```python
from build123d import *

# Parameters (mm, degrees)
SKETCH1_W           = 175.26
SKETCH1_H           = 12.7
BOSS_EXTRUDE1_DEPTH = 98.425
SKETCH2_W           = 5.08
SKETCH2_H           = 6.35
CUT_EXTRUDE1_DEPTH  = 216.567302483
CUT_EXTRUDE2_DEPTH  = 133.392550867
CUT_EXTRUDE3_DEPTH  = 133.392550867


with BuildPart() as part:
    # Sketch1 → Boss-Extrude1 (new, symmetric)
    with BuildSketch(Plane(origin=(0, 0, 0), x_dir=(0, 0, -1), z_dir=(1, 0, 0))):
        Rectangle(SKETCH1_W, SKETCH1_H)
    extrude(amount=BOSS_EXTRUDE1_DEPTH, both=True)

    # Sketch2 → Cut-Extrude1 (cut, through all)
    with BuildSketch(Plane(origin=(98.425, 0, 0), x_dir=(0, 0, -1), z_dir=(1, 0, 0))):
        with Locations((-85.09, -3.175)):
            Rectangle(SKETCH2_W, SKETCH2_H)
        with Locations((85.09, -3.175)):
            Rectangle(SKETCH2_W, SKETCH2_H)
    extrude(amount=-CUT_EXTRUDE1_DEPTH, mode=Mode.SUBTRACT)

    # Sketch3 → Cut-Extrude2 (cut, through all)
    with BuildSketch(Plane(origin=(0, 6.35, 0), x_dir=(1, 0, 0), z_dir=(0, 1, 0))):
        with BuildLine():
            Line((28.448, -41.148), (41.402, -41.148))
            ThreePointArc((41.402, -41.148), (44.704, -44.45), (41.402, -47.752))
            Line((41.402, -47.752), (41.402, -57.023))
            ThreePointArc((41.402, -57.023), (44.704, -60.325), (41.402, -63.627))
            Line((41.402, -63.627), (28.448, -63.627))
            ThreePointArc((28.448, -63.627), (25.146, -60.325), (28.448, -57.023))
            Line((28.448, -57.023), (28.448, -47.752))
            ThreePointArc((28.448, -47.752), (25.146, -44.45), (28.448, -41.148))
        make_face()
        with BuildLine():
            Line((-22.352, -41.148), (-9.398, -41.148))
            ThreePointArc((-9.398, -41.148), (-6.096, -44.45), (-9.398, -47.752))
            Line((-9.398, -47.752), (-9.398, -57.023))
            ThreePointArc((-9.398, -57.023), (-6.096, -60.325), (-9.398, -63.627))
            Line((-9.398, -63.627), (-22.352, -63.627))
            ThreePointArc((-22.352, -63.627), (-25.654, -60.325), (-22.352, -57.023))
            Line((-22.352, -57.023), (-22.352, -47.752))
            ThreePointArc((-22.352, -47.752), (-25.654, -44.45), (-22.352, -41.148))
        make_face()
        with BuildLine():
            Line((-22.352, 63.627), (-9.398, 63.627))
            ThreePointArc((-9.398, 63.627), (-6.096, 60.325), (-9.398, 57.023))
            Line((-9.398, 57.023), (-9.398, 47.752))
            ThreePointArc((-9.398, 47.752), (-6.096, 44.45), (-9.398, 41.148))
            Line((-9.398, 41.148), (-22.352, 41.148))
            ThreePointArc((-22.352, 41.148), (-25.654, 44.45), (-22.352, 47.752))
            Line((-22.352, 47.752), (-22.352, 57.023))
            ThreePointArc((-22.352, 57.023), (-25.654, 60.325), (-22.352, 63.627))
        make_face()
        with BuildLine():
            Line((28.448, 63.627), (41.402, 63.627))
            ThreePointArc((41.402, 63.627), (44.704, 60.325), (41.402, 57.023))
            Line((41.402, 57.023), (41.402, 47.752))
            ThreePointArc((41.402, 47.752), (44.704, 44.45), (41.402, 41.148))
            Line((41.402, 41.148), (28.448, 41.148))
            ThreePointArc((28.448, 41.148), (25.146, 44.45), (28.448, 47.752))
            Line((28.448, 47.752), (28.448, 57.023))
            ThreePointArc((28.448, 57.023), (25.146, 60.325), (28.448, 63.627))
        make_face()
    extrude(amount=-CUT_EXTRUDE2_DEPTH, mode=Mode.SUBTRACT)

    # Sketch4 → Cut-Extrude3 (cut, through all)
    with BuildSketch(Plane(origin=(0, 6.35, 0), x_dir=(1, 0, 0), z_dir=(0, 1, 0))):
        with BuildLine():
            Line((55.5625, -68.2625), (55.5625, -23.8125))
            ThreePointArc((55.5625, -23.8125), (60.325, -19.05), (65.0875, -23.8125))
            Line((65.0875, -23.8125), (65.0875, -68.2625))
            ThreePointArc((65.0875, -68.2625), (60.325, -73.025), (55.5625, -68.2625))
        make_face()
        with BuildLine():
            Line((55.5625, 23.8125), (55.5625, 68.2625))
            ThreePointArc((55.5625, 68.2625), (60.325, 73.025), (65.0875, 68.2625))
            Line((65.0875, 68.2625), (65.0875, 23.8125))
            ThreePointArc((65.0875, 23.8125), (60.325, 19.05), (55.5625, 23.8125))
        make_face()
        with BuildLine():
            Line((84.1375, 68.2625), (84.1375, 23.8125))
            ThreePointArc((84.1375, 23.8125), (79.375, 19.05), (74.6125, 23.8125))
            Line((74.6125, 23.8125), (74.6125, 68.2625))
            ThreePointArc((74.6125, 68.2625), (79.375, 73.025), (84.1375, 68.2625))
        make_face()
        with BuildLine():
            Line((84.1375, -23.8125), (84.1375, -68.2625))
            ThreePointArc((84.1375, -68.2625), (79.375, -73.025), (74.6125, -68.2625))
            Line((74.6125, -68.2625), (74.6125, -23.8125))
            ThreePointArc((74.6125, -23.8125), (79.375, -19.05), (84.1375, -23.8125))
        make_face()
    extrude(amount=-CUT_EXTRUDE3_DEPTH, mode=Mode.SUBTRACT)


solid = part.part
```
The model under review builds one solid part; all positions refer to its coordinate system, in mm. A direction names the side the tool comes from. Coordinates: 2 decimals unless noted, no trailing zeros. Write each loop counter-clockwise with the first axis right and the second up, starting at its lowest first coordinate (ties: lowest second). Pieces come first, ordered by that corner, then holes.
1) We need section B-B on x = -56. State the section outline as (y, z) points.
2) We need section A-A on z = -44.45. Count the separate pieces of the cut face and the enclosed holes in it, then the cut area to 3 significant figures.
3) The part is to be moulded in two halves that separate along X. For faces 1 (the face through (79.48, 0.089, 73.024)), 2 (the face through (1, -6.35, 1)), 3 (the face through (98.425, 0, 1)), say which applies: pulls with the +X half, pulls with the -X half, needs draft (parallel to the pull), parting line crosses it, or undercut.
4) Machinability: for faces 4 (the face through (74.612, 0, -46)), 5 (the face through (1, 3, 87.63)), 6 (the face through (1, -3, 82.55)), which of the approach directions +Z, -Z, +X, -X, +Y, -Y give a long, thin tool a straight path to every point of the face, cutting with its end or side? Answer none if there is none.
5) Clearance check with flat-ended pins moving along their axes: pin 1 Ø3 at (x, y) = (36, -3) entering from +Z; pin 2 Ø6.5 at (x, y) = (33, -0.5) entering from -Z; pin 3 Ø2 at (x, y) = (-11, -2) entering from -Z; pin 4 Ø2.5 at (x, z) = (43, -85.5) entering from -Y. State where each tip first meets the part, or that it passes through.
6) To check wall thickness, follow probe 1 along X at (y, z) = (0, 36) (1 decimal); probe 2 along X at (y, z) = (5.5, -50) (1 decimal); probe 3 along Z at (x, y) = (43.5, -2). State the ranges of each line that lie inside material, in increasing order.
Answer list:
1. outline: (-6.35, -82.55) - (0, -82.55) - (0, -87.63) - (6.35, -87.63) - (6.35, 87.63) - (0, 87.63) - (0, 82.55) - (-6.35, 82.55) - close
2. separate pieces: 5
2. enclosed holes: 0
2. area: 1,760 mm2
3. face 1: undercut
3. face 2: needs draft
3. face 3: pulls with the +X half
4. face 4: +Y, -Y
4. face 5: +Z, +X, -X, +Y, -Y
4. face 6: +Z, +X, -X, -Y
5. pin 1: stops at z = 82.55
5. pin 2: stops at z = -87.63
5. pin 3: stops at z = -82.55
5. pin 4: stops at y = 0
6. probe 1: x = -98.4 to 55.6, 65.1 to 74.6, 84.1 to 98.4
6. probe 2: x = -98.4 to -22.4, -9.4 to 28.4, 41.4 to 55.6, 65.1 to 74.6, 84.1 to 98.4
6. probe 3: z = -82.55 to -62.87, -57.78 to -47, -41.9 to 41.9, 47 to 57.78, 62.87 to 82.55
